from build123d import *

# Parameters (mm, degrees)
SKETCH_1_R          = 84
EXTRUDE_1_DEPTH     = 2
SKETCH_2_R          = 1.5
CUT_EXTRUDE_1_DEPTH = 2
SKETCH_3_R          = 15
SKETCH_3_R_2        = 22.5
CUT_EXTRUDE_2_DEPTH = 2
SKETCH_4_R          = 20
CUT_EXTRUDE_3_DEPTH = 1


with BuildPart() as part:
    # 草图1 → 凸台-拉伸1 (new body)
    with BuildSketch(Plane(origin=(0, 0, 0), x_dir=(1, 0, 0), z_dir=(0, 1, 0))):
        with Locations(Location((0, 0, 0), (0, 0, 270))):
            Circle(SKETCH_1_R)
    extrude(amount=EXTRUDE_1_DEPTH)

    # 草图2 → 切除-拉伸1 (cut)
    with BuildSketch(Plane(origin=(0, 2, 0), x_dir=(1, 0, 0), z_dir=(0, 1, 0))):
        with Locations(Location((0, 80, 0), (0, 0, 270))):
            Circle(SKETCH_2_R)
        with Locations(Location((56.568542495, 56.568542495, 0), (0, 0, 270))):
            Circle(SKETCH_2_R)
        with Locations(Location((80, 0, 0), (0, 0, 270))):
            Circle(SKETCH_2_R)
        with Locations(Location((56.568542495, -56.568542495, 0), (0, 0, 270))):
            Circle(SKETCH_2_R)
        with Locations(Location((0, -80, 0), (0, 0, 270))):
            Circle(SKETCH_2_R)
        with Locations(Location((-56.568542495, -56.568542495, 0), (0, 0, 270))):
            Circle(SKETCH_2_R)
        with Locations(Location((-80, 0, 0), (0, 0, 270))):
            Circle(SKETCH_2_R)
        with Locations(Location((-56.568542495, 56.568542495, 0), (0, 0, 270))):
            Circle(SKETCH_2_R)
    extrude(amount=-CUT_EXTRUDE_1_DEPTH, mode=Mode.SUBTRACT)

    # 草图3 → 切除-拉伸2 (cut)
    with BuildSketch(Plane(origin=(0, 2, 0), x_dir=(1, 0, 0), z_dir=(0, 1, 0))):
        with Locations(Location((-25, 0, 0), (0, 0, 270))):
            Circle(SKETCH_3_R)
        with Locations(Location((40, 0, 0), (0, 0, 270))):
            Circle(SKETCH_3_R_2)
    extrude(amount=-CUT_EXTRUDE_2_DEPTH, mode=Mode.SUBTRACT)

    # 草图4 → 切除-拉伸3 (cut)
    with BuildSketch(Plane(origin=(0, 2, 0), x_dir=(1, 0, 0), z_dir=(0, 1, 0))):
        with Locations(Location((-25, 0, 0), (0, 0, 270))):
            Circle(SKETCH_4_R)
    extrude(amount=-CUT_EXTRUDE_3_DEPTH, mode=Mode.SUBTRACT)

    # 草图6 → 旋转1 (revolve)
    with BuildSketch(Plane.XY):
        Polygon((0, 2), (17.5, 2), (27.498489886, -7.998489886), (34.998489886, -7.998489886), (34.998489886, -8.998489886), (37.498489886, -8.998489886), (37.498489886, -9.998489886), (26.088489886, -9.998489886), (16.09, 0), (0, 0), align=None)
    revolve(axis=Axis((40, 0, 0), (0, -1, 0)))


solid = part.part
Read the model definition and answer for the solid it produces. Units are mm, in the model's axes. A direction names the side the tool comes from. Give positions to 0.01 mm unless a question says otherwise; leave off trailing zeros. Loops run counter-clockwise (first coordinate to the right, second up) from the corner with the lowest first, then second, coordinate; pieces in that order, holes last. Notation, with made-up numbers: (-18.5, 77) -> (36.5, 77) arc R18 cw to (36.5, 110) -> close; hole circle Ø3 at (-32, 19.25). An arc over 180 degrees is marked (long way). Answer as CSV lines item,"result".
Item 1: For faces 1 (the face through (-39.643, 0.507, -3.252)), 2 (the face through (-10, 1, 3)), determine the directions among +Z, -Z, +X, -X, +Y, -Y from which every point of the face is accessible in a straight line to the end or side of a thin tool.
Returned:
face 1,"+Y, -Y"
face 2,"+Y"
Item 2: Determine the mould class of faces 3 (the face through (25.23, 0.99, 80.12)), 4 (the face through (38, -8.998, 2)), 5 (the face through (1, 2, -1)) for opening direction X: +X half, -X half, draft (parallel to the pull), parting line (faces both ways), or undercut.
Returned:
face 3,"parting line"
face 4,"undercut"
face 5,"draft"
Item 3: Each of these flat-tipped pins is pushed along its axis until it touches: pin 1 (1.5 mm diameter, centred on x = -5, z = -25, fed in from -Y); pin 2 (8 mm diameter, centred on x = 39.5, z = -1, fed in from +Y). Where does it stop, or does it pass through?
Returned:
pin 1,"stops at y = 0"
pin 2,"stops at y = -8"
Item 4: Consider line 1 (Y direction, x = -7, z = 59.5); line 2 (X direction, y = -8.3, z = 0); line 3 (Y direction, x = 47, z = -1). Determine where each line is inside the solid, lowest interval first. Write a range as [from, to].
Returned:
line 1,"y = [0, 2]"
line 2,"x = [24.39, 35], [45, 55.61]"
line 3,"y = [-10, -8]"
Item 5: Find section B-B on y = -2.75. Give the vertices of the cut face in (x, z), plus the area to 3 significant figures.
Returned:
outline,"circle Ø42.32 at (40, 0); hole circle Ø35.5 at (40, 0)"
area,"417 mm²"
Item 6: Find section D-D on z = -60. Give the vertices of the cut face in (x, y), plus the area to 3 significant figures.
Returned:
outline,"(-58.79, 0) -> (58.79, 0) -> (58.79, 2) -> (-58.79, 2) -> close"
area,"235 mm²"
Item 7: Find section A-A on x = 40. Give the vertices of the cut face in (y, z), plus the area to 3 significant figures.
Returned:
outline,"(-10, -13.91) -> (0, -23.91) -> (0, -73.86) -> (2, -73.86) -> (2, -22.5) -> (-8, -12.5) -> (-8, -5) -> (-9, -5) -> (-9, -2.5) -> (-10, -2.5) -> close; (-10, 2.5) -> (-9, 2.5) -> (-9, 5) -> (-8, 5) -> (-8, 12.5) -> (2, 22.5) -> (2, 73.86) -> (0, 73.86) -> (0, 23.91) -> (-10, 13.91) -> close"
area,"309 mm²"
Item 8: Find section C-C on x = -25. Give the vertices of the cut face in (y, z), plus the area to 3 significant figures.
Returned:
outline,"(0, -80.19) -> (2, -80.19) -> (2, -20) -> (1, -20) -> (1, -15) -> (0, -15) -> close; (0, 15) -> (1, 15) -> (1, 20) -> (2, 20) -> (2, 80.19) -> (0, 80.19) -> close"
area,"251 mm²"
